Could you check a few things on this drawing? It's one solid part, dimensions in mm from its lowest x, y, z. Give positions to 0.01 mm unless a question says otherwise; leave off trailing zeros. Loops run counter-clockwise (first coordinate to the right, second up) from the corner with the lowest first, then second, coordinate; pieces in that order, holes last. Notation, with made-up numbers: (22.5, 36) -> (77.5, 36) arc R13 cw to (77.5, 51) -> close; hole circle Ø4 at (47, -39.75). An arc over 180 degrees is marked (long way). Use CSV: the item, a comma, the result in double quotes.
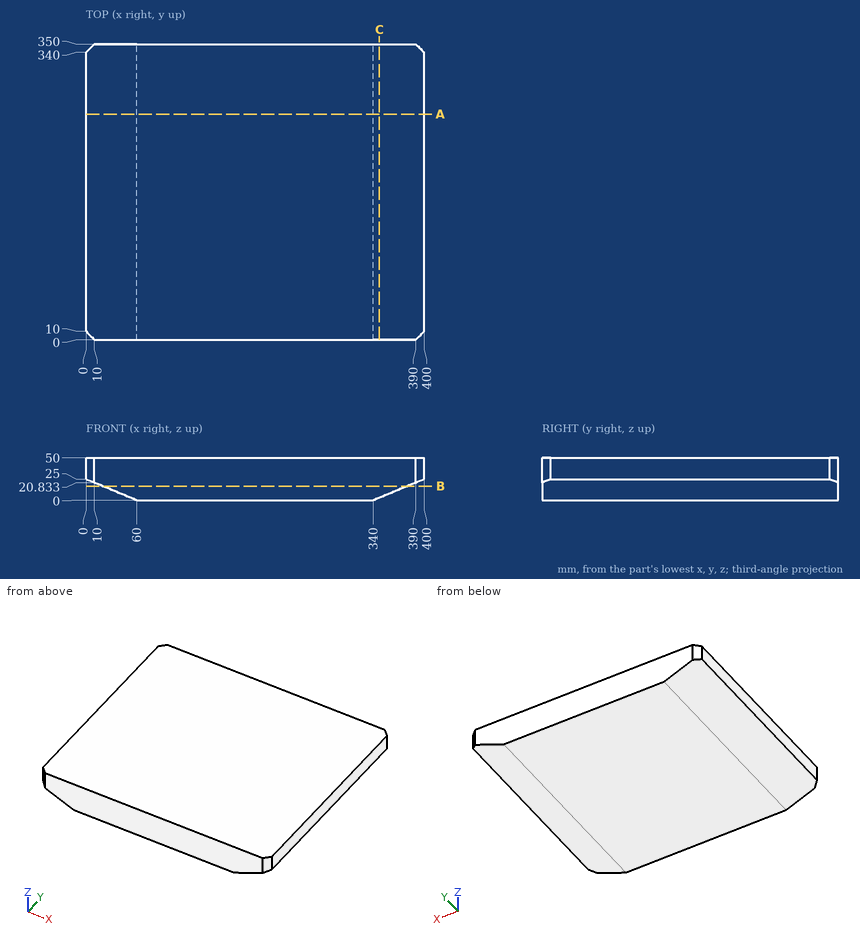
(1) Will these pins go through, and if not, where does the flat tip stop? pin 1 Ø6 at (y, z) = (260, 17) entering from -X; pin 2 Ø2 at (y, z) = (207, 16.5) entering from -X; pin 3 Ø6 at (y, z) = (112, 18) entering from -X.
Answer sheet:
pin 1,"stops at x = 12"
pin 2,"stops at x = 18"
pin 3,"stops at x = 9.6"
(2) If we section it at B-B, the plane z = 16.5: Write out the boundary of the cut face in (x, y).
Answer sheet:
outline,"(20.4, 0) -> (379.6, 0) -> (379.6, 350) -> (20.4, 350) -> close"
(3) If we section it at A-A, the plane y = 267: Write out the boundary of the cut face in (x, z), then the cut area to 3 significant figures.
Answer sheet:
outline,"(0, 25) -> (60, 0) -> (340, 0) -> (400, 25) -> (400, 50) -> (0, 50) -> close"
area,"18,500 mm2"
(4) If I drill on L1, parallel to Z at x = 364, y = 59; L2, parallel to X at y = 15.5, z = 16.5; L3, parallel to X at y = 183, z = 5.5, over which ranges is the centre line in solid material (lowest first)? Write a range as from..to.
Answer sheet:
L1,"z = 10..50"
L2,"x = 20.4..379.6"
L3,"x = 46.8..353.2"
(5) If we section it at C-C, the plane x = 347: Write out the boundary of the cut face in (y, z), then the cut area to 3 significant figures.
Answer sheet:
outline,"(0, 2.92) -> (350, 2.92) -> (350, 50) -> (0, 50) -> close"
area,"16,500 mm2"
